Autodesk Inventor part; units mm, degrees
ref_plane "YZ Plane" through (0, 0, 0) normal (1, 0, 0) x (0, 1, 0)
ref_plane "XZ Plane" through (0, 0, 0) normal (0, 1, 0) x (-1, 0, 0)
ref_plane "XY Plane" through (0, 0, 0) normal (0, 0, 1) x (1, 0, 0)
sketch "スケッチ1" plane through (0, 0, 0) normal (0, 0, 1) x (1, 0, 0)
  circle A0 centre (0, 0) radius 10.5 construction
  line L0 (0, 10.5) -> (-162.5, 10.5) construction
  line L1 (-162.5, 10.5) -> (-162.5, -10.5) construction
  line L2 (-162.5, -10.5) -> (0, -10.5) construction
  circle A1 centre (-157.5, 0) radius 1.55
  line L3 (-147.5, 2.5) -> (-32.5, 2.5) construction
  line L4 (-32.5, 2.5) -> (-32.5, -2.5) construction
  line L5 (-32.5, -2.5) -> (-147.5, -2.5) construction
  line L6 (-147.5, -2.5) -> (-147.5, 2.5) construction
  line L7 (-90, 2.5) -> (-90, -2.5) construction
  circle A2 centre (-22.5, 0) radius 1.55
  line L8 (-12, 21.3027) -> (-12, -27.3903) construction
  line L9 (-32.45, 2.55) -> (-147.55, 2.55) construction
  line L10 (-147.55, 2.55) -> (-147.55, -2.55) construction
  line L11 (-147.55, -2.55) -> (-32.45, -2.55) construction
  line L12 (-32.45, -2.55) -> (-32.45, 2.55) construction
  circle A3 centre (-146.5, 2.55) radius 1.05 construction
  line L13 (-147.5, 0) -> (-90, 0) construction
  line L14 (-147.55, 2.55) -> (-147.55, -2.55)
  arc A4 (-145.45, 2.55) -> (-147.55, 2.55) centre (-146.5, 2.55) ccw
  line L15 (-145.45, 2.55) -> (-34.55, 2.55)
  arc A5 (-32.45, 2.55) -> (-34.55, 2.55) centre (-33.5, 2.55) ccw
  line L16 (-32.45, 2.55) -> (-32.45, -2.55)
  arc A6 (-147.55, -2.55) -> (-145.45, -2.55) centre (-146.5, -2.55) ccw
  line L17 (-145.45, -2.55) -> (-34.55, -2.55)
  arc A7 (-34.55, -2.55) -> (-32.45, -2.55) centre (-33.5, -2.55) ccw
  circle A8 centre (0, 8.5) radius 1.35
  circle A9 centre (0, 0) radius 5.05
  circle A10 centre (-8.5, 0) radius 1.35
  circle A11 centre (0, -8.5) radius 1.35
  circle A12 centre (8.5, 0) radius 1.35
  line L18 (-162.5, 4.8006) -> (-162.5, -4.8006)
  line L19 (-162.5, 4.8006) -> (-22.5, 10.5)
  line L20 (-22.5, 10.5) -> (0, 10.5)
  line L21 (-162.5, -4.8006) -> (-22.5, -10.5)
  line L22 (-22.5, -10.5) -> (0, -10.5)
  arc A13 (0, -10.5) -> (0, 10.5) centre (0, 0) ccw
  circle A14 centre (-157.5, 0) radius 5 construction
  point P0 (-162.5, 0)
  dimension "d9" = 2.1
  dimension "d0" = 162.5
  dimension "d1" = 3.1
  dimension "d2" = 21
  dimension "d3" = 10
  dimension "d4" = 5
  dimension "d5" = 12
  dimension "d6" = 135
  dimension "d7" = 5
  dimension "d8" = 0.05
  dimension "d10" = 2.7
  dimension "d11" = 8.5
  dimension "d12" = 10.1
  dimension "d15" = 360
extrude "押し出し1" add sketch "スケッチ1" along normal blind 2
fillet "フィレット1" radius 2 2 edges at (-162.5, -4.8006, 1) (-162.5, 4.8006, 1)
sketch "スケッチ2" plane through (0, 0, 0) normal (0, 0, -1) x (-1, 0, 0)
  circle A0 centre (22.5, 0) radius 1.55
  circle A1 centre (22.5, 0) radius 1.55
  circle A2 centre (8.5, 0) radius 1.35
  circle A3 centre (8.5, 0) radius 1.35
  circle A4 centre (0, -8.5) radius 1.35
  circle A5 centre (0, -8.5) radius 1.35
  circle A6 centre (-8.5, 0) radius 1.35
  circle A7 centre (-8.5, 0) radius 1.35
  circle A8 centre (0, 8.5) radius 1.35
  circle A9 centre (0, 8.5) radius 1.35
  circle A10 centre (157.5, 0) radius 1.55
  circle A11 centre (157.5, 0) radius 1.55
  point P0 (0, 0)
extrude "押し出し2" add sketch "スケッチ2" against normal up to surface (2 mm away)
equation "\"H_head\" = 28.5"
equation "\"H_leg\" = 199.5"
equation "\"足の面積\" = 12720.125"
equation "\"現在の面積\" = 11560"
equation "\"足_短辺\" = 68"
equation "\"円柱\" = 313.5"
equation "\"胴体中心から手先\" = 342"
equation "\"H_leg_1\" = 186.2"
equation "\"H_leg_MAX\" = 399"
equation "\"H_head_1\" = 26.6"
equation "\"H_head_MAX\" = 142.5"
properties part number "前腕_メインフレーム_1_1" material "GFRP"
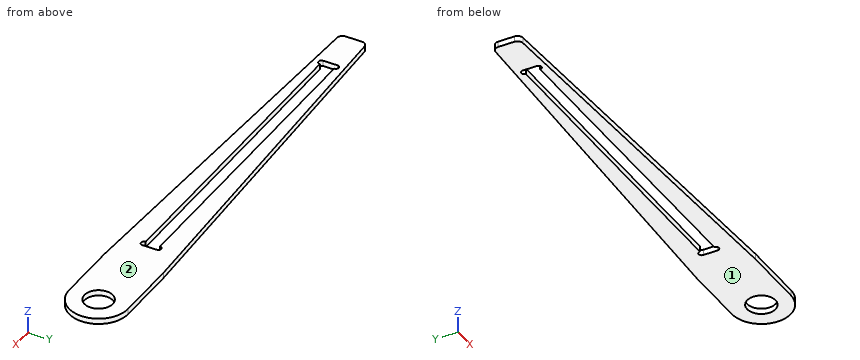
Input: part model. Units: mm. Frame: model coordinates. Face numbers are marked on the shaded views. Give positions to 0.01 mm unless a question says otherwise; leave off trailing zeros. Order: outer loops, then holes, each group sorted by start corner. A loop starts at its lowest first (then second) coordinate and runs counter-clockwise, first axis right, second up. Notation, with made-up numbers: M 76.5,-7.5 L 113.5,-7.5 A22 cw 113.5,28.5 Z; hole C 30,64 d10. An arc over 180 degrees is marked long. Return JSON: item names as keys, results as strings.
Item 1: Cut plane B-B (x = -52.5). Return loops of the section in (y, z), then the cut area to 3 significant figures.
Solutions:
{"outline": "M -9.28,0 L -2.55,0 L -2.55,2 L -9.28,2 Z; M 2.55,0 L 9.28,0 L 9.28,2 L 2.55,2 Z", "area": "26.9 mm^2"}
Item 2: First-contact query: P1, Ø1, axis at y = -3.5, z = 1.5, coming from the -X side; P2, Ø0.6, axis at y = -0.5, z = 1, coming from the +X side; P3, Ø0.6, axis at x = -85, z = 1, coming from the +Y side; P4, Ø2, axis at x = -126, y = 3, coming from the -Z side. Flat tips, straight axial feed; report the tip coordinate or a pass-through.
Solutions:
{"P1": "x = -162.5", "P2": "x = 10.5", "P3": "y = 7.97", "P4": "z = 0"}
Item 3: Cut plane C-C (x = -104). Return loops of the section in (y, z), then the cut area to 3 significant figures.
Solutions:
{"outline": "M -7.18,0 L -2.55,0 L -2.55,2 L -7.18,2 Z; M 2.55,0 L 7.18,0 L 7.18,2 L 2.55,2 Z", "area": "18.5 mm^2"}
Item 4: Cut plane D-D (y = -8.25). Return loops of the section in (x, z), then the cut area to 3 significant figures.
Solutions:
{"outline": "M -77.77,0 L 6.5,0 L 6.5,2 L -77.77,2 Z", "area": "169 mm^2"}
Item 5: Pull-direction query (Z, two-part tool) for the marked faces 1 and 2; classes: +Z half, -Z half, draft (parallel to the pull), parting line (faces both ways), or undercut.
Solutions:
{"face 1": "-Z half", "face 2": "+Z half"}
Item 6: Ray query, probe 1 along X at (y, z) = (-0.25, 1.1); probe 2 along Y at (x, z) = (0, 0.45); probe 3 along X at (y, z) = (2.25, 0.2). Return the intervals inside material, ascending.
Solutions:
{"probe 1": "-162.5 to -147.55, -32.45 to -5.04, 5.04 to 10.5", "probe 2": "-10.5 to -5.05, 5.05 to 10.5", "probe 3": "-162.5 to -147.55, -32.45 to -4.52, 4.52 to 10.26"}
Item 7: Cut plane A-A (z = 0.5). Return loops of the section in (x, y).
Solutions:
{"outline": "M -162.5,-2.88 A2 ccw -160.58,-4.88 L -22.5,-10.5 L 0,-10.5 A10.5 ccw 0,10.5 L -22.5,10.5 L -160.58,4.88 A2 ccw -162.5,2.88 Z; hole M -147.55,-2.55 A1.05 ccw -145.45,-2.55 L -34.55,-2.55 A1.05 ccw -32.45,-2.55 L -32.45,2.55 A1.05 ccw -34.55,2.55 L -145.45,2.55 A1.05 ccw -147.55,2.55 Z; hole C 0,0 d10.1"}
